Drawing for the job (mm, zero at the part's lowest x, y, z). A direction names the side the tool comes from. Coordinates: 2 decimals unless noted, no trailing zeros. Loops run counter-clockwise (first coordinate to the right, second up) from the corner with the lowest first, then second, coordinate; pieces in that order, holes last.
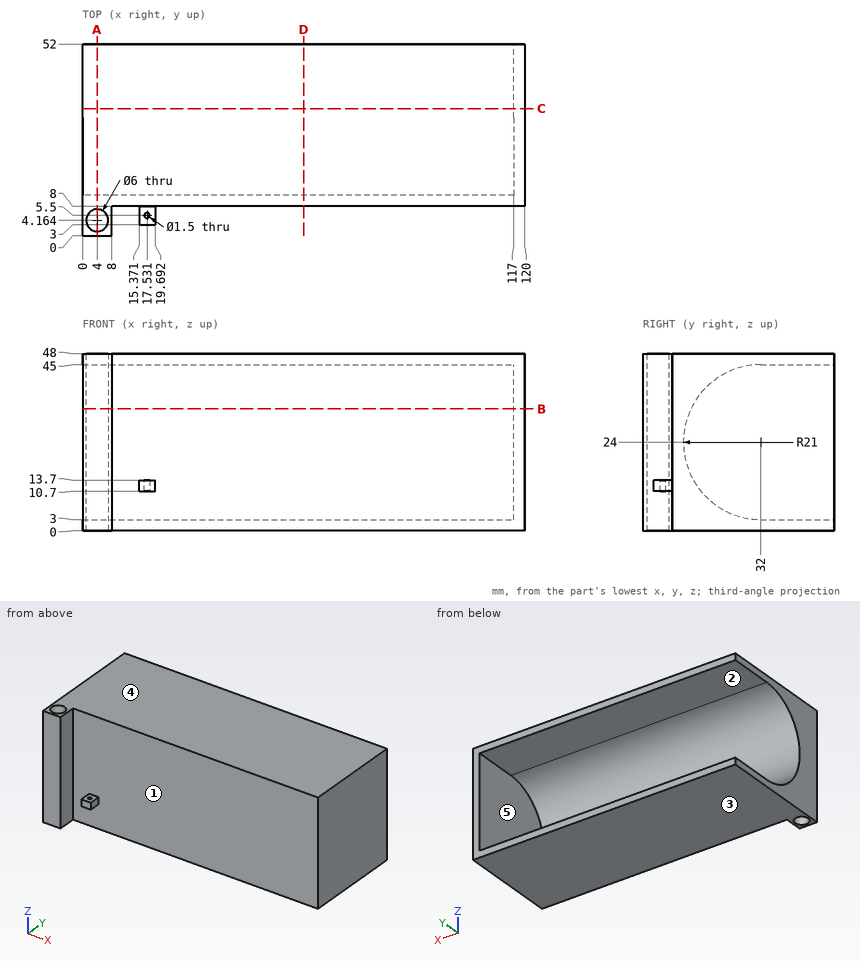
Q1. Tool access for the marked faces 4 and 5: list every direction of +Z, -Z, +X, -X, +Y, -Y with a clear straight run to the whole face (end or side of a thin tool).
Q2. Saw through at C-C (y = 34.5). List the corners of the cut face in (x, z).
Q3. Probe line 1 (X direction, y = 5, z = 11); line 2 (X direction, y = 5.5, z = 12.1) (1 decimal); line 3 (X direction, y = 32, z = 15.5). List the from-to ranges inside material, lowest first.
Q4. Drop flat-ended pins along their axis: P1, Ø0.9, axis at y = 5, z = 13, coming from the -X side; P2, Ø2.5, axis at y = 5, z = 12, coming from the +X side; P3, Ø3, axis at x = 60.5, z = 33, coming from the -Y side; P4, Ø1.3, axis at x = 18, y = 6, coming from the +Z side. Give the stop position or say it passes through.
Q5. Saw through at B-B (z = 33). List the corners of the cut face in (x, y) (1 decimal).
Q6. Saw through at A-A (x = 4). List the corners of the cut face in (y, z) (1 decimal).
Q7. Mould opens along Z. For the marked faces 1, 2 and 3 say: released by +Z, released by -Z, zero draft, split by the parting line, or undercut.
Q8. Saw through at D-D (x = 60). List the corners of the cut face in (y, z).
Checked values:
1. face 4: +Z, +X, -X, +Y, -Y
1. face 5: -X, +Y
2. outline: (0, 0) - (120, 0) - (120, 48) - (0, 48) - (0, 45) - (117, 45) - (117, 3) - (0, 3) - close
3. line 1: x = 0 to 1.12, 6.88 to 8, 15.37 to 16.97, 18.09 to 19.69
3. line 2: x = 0 to 1.3, 6.7 to 8, 15.4 to 16.8, 18.3 to 19.7
3. line 3: x = 117 to 120
4. P1: stops at x = 0
4. P2: stops at x = 19.69
4. P3: stops at y = 8
4. P4: stops at z = 13.7
5. outline: (0, 0) - (8, 0) - (8, 8) - (120, 8) - (120, 52) - (117, 52) - (117, 13) - (0, 13) - close; hole circle Ø6 at (4, 4.2)
6. outline: (0, 0) - (1.2, 0) - (1.2, 48) - (0, 48) - close; (7.2, 0) - (52, 0) - (52, 3) - (32, 3) arc R21 cw to (32, 45) - (52, 45) - (52, 48) - (7.2, 48) - close
7. face 1: zero draft
7. face 2: undercut
7. face 3: released by -Z
8. outline: (8, 0) - (52, 0) - (52, 3) - (32, 3) arc R21 cw to (32, 45) - (52, 45) - (52, 48) - (8, 48) - close
